Part model, mm, in its own coordinate system. A direction names the side the tool comes from. Give positions to 0.01 mm unless a question says otherwise; leave off trailing zeros. Write each loop counter-clockwise with the first axis right and the second up, starting at its lowest first coordinate (ties: lowest second). Pieces come first, ordered by that corner, then holes.
```python
from build123d import *

# Parameters (mm, degrees)
F0_R     = 7.5
F1_DEPTH = 60
F3_DEPTH = 30.001
F4_W     = 40
F4_H     = 22
F5_DEPTH = 30.001
F6_R     = 17
F6_R_2   = 10
F7_DEPTH = 13
F8_R     = 10
F9_DEPTH = 47.001


with BuildPart() as f1:
    # F0 (on Right) → F1 (new body)
    with BuildSketch(Plane.YZ):
        with BuildLine():
            Line((-15, 10), (-15, 0))
            Line((-15, 0), (15, 0))
            Line((15, 0), (15, 10))
            Line((15, 10), (15, 32))
            ThreePointArc((15, 32), (0, 47), (-15, 32))
            Line((-15, 32), (-15, 10))
        make_face()
        with Locations((0, 32)):
            Circle(F0_R, mode=Mode.SUBTRACT)
    extrude(amount=F1_DEPTH)

    # F2 (on face) → F3 (cut, through all)
    with BuildSketch(Plane.XZ.offset(15)):
        Polygon((50, 85.158385), (10, 82.922354), (10, 32), (50, 32), align=None)
    extrude(amount=-F3_DEPTH, mode=Mode.SUBTRACT)

    # F4 (on face) → F5 (cut, through all)
    with BuildSketch(Plane.XZ.offset(15)):
        with Locations((30, 21)):
            Rectangle(F4_W, F4_H)
    extrude(amount=-F5_DEPTH, mode=Mode.SUBTRACT)

    # F6 (on face) → F7 (join)
    with BuildSketch(Plane.XY.offset(10)):
        with Locations((30, 0)):
            Circle(F6_R)
        with Locations((30, 0)):
            Circle(F6_R_2, mode=Mode.SUBTRACT)
    extrude(amount=-F7_DEPTH)

    # F8 (on face) → F9 (cut, through all)
    with BuildSketch(Plane(origin=(0, 0, 0), x_dir=(1, 0, 0), z_dir=(0, 0, -1))):
        with Locations((30, 0)):
            Circle(F8_R)
    extrude(amount=-F9_DEPTH, mode=Mode.SUBTRACT)


solid = f1.part
```
1) Saw through at D-D, the plane x = 30. Write the cut outline in (y, z).
Answers follow:
outline: (-17, -3) - (-10, -3) - (-10, 10) - (-17, 10) - close; (10, -3) - (17, -3) - (17, 10) - (10, 10) - close
2) Saw through at B-B, the plane y = 0. Write the cut outline in (x, z).
Answers follow:
outline: (0, 0) - (13, 0) - (13, -3) - (20, -3) - (20, 10) - (10, 10) - (10, 24.5) - (0, 24.5) - close; (0, 39.5) - (10, 39.5) - (10, 47) - (0, 47) - close; (40, -3) - (47, -3) - (47, 0) - (60, 0) - (60, 24.5) - (50, 24.5) - (50, 10) - (40, 10) - close; (50, 39.5) - (60, 39.5) - (60, 47) - (50, 47) - close
3) Wall check: L1, parallel to X at y = 7.5, z = 14; L2, parallel to Y at x = 30, z = 0; L3, parallel to Z at x = 52, y = 0. Give the ranges that are in metal, low to high.
Answers follow:
L1: x = 0 to 10, 50 to 60
L2: y = -17 to -10, 10 to 17
L3: z = 0 to 24.5, 39.5 to 47
4) 3-axis set-ups, long thin cutter, end or side, ignore diameter. For faces 4 (the face through (51, -15, 13)), 5 (the face through (51, 15, 12)), 6 (the face through (37.844, -15.082, 2.147)): which of +Z, -Z, +X, -X, +Y, -Y reach the whole face in a straight line?
Answers follow:
face 4: +Z, -Z, +X, -Y
face 5: +Z, -Z, +X, +Y
face 6: -Z
5) Two-plate mould, pull along Z, no slides. Class faces 1 (the face through (30, 11, 10)), 2 (the face through (4.93, -1.63, 24.68)), 3 (the face through (10, 0, 24)): +Z half, -Z half, draft (parallel to the pull), parting line (faces both ways), or undercut.
Answers follow:
face 1: +Z half
face 2: undercut
face 3: draft
6) Pin check, flat tips, straight feed: pin 1 Ø18 at (x, y) = (30, 0) entering from +Z; pin 2 Ø6.5 at (x, z) = (47, 18) entering from +Y; pin 3 Ø11 at (x, z) = (6, 16) entering from -Y; pin 4 Ø12 at (x, y) = (7.5, -11) entering from -Z. Stop position of each tip, or through.
Answers follow:
pin 1: passes through
pin 2: stops at y = 15
pin 3: stops at y = -15
pin 4: stops at z = 0
7) Saw through at A-A, the plane x = 8. Write the cut outline in (y, z), then the cut area to 3 significant figures.
Answers follow:
outline: (-15, 0) - (15, 0) - (15, 32) arc R15 ccw to (-15, 32) - close; hole circle Ø15 at (0, 32)
area: 1,140 mm2
8) Saw through at C-C, the plane z = 5. Write the cut outline in (x, y).
Answers follow:
outline: (0, -15) - (22, -15) arc R17 ccw to (38, -15) - (60, -15) - (60, 15) - (38, 15) arc R17 ccw to (22, 15) - (0, 15) - close; hole circle Ø20 at (30, 0)
